Build history of the part. All positions in model axes, mm. A direction names the side the tool comes from. Round coordinates to 2 decimals unless told otherwise and drop trailing zeros. Write each loop counter-clockwise with the first axis right and the second up, starting at its lowest first coordinate (ties: lowest second). Pieces come first, ordered by that corner, then holes.
Item 1: Wall check: probe 1 along X at (y, z) = (0, 5.75); probe 2 along Y at (x, z) = (-60, 25.5); probe 3 along Z at (x, y) = (30, -40.5). Give the ranges that are in metal, low to high.
Item 2: Mould opens along Y. For faces 1 (the flat face through (6.5, -0.2, 10)), 2 (the flat face through (-80, 0, 15)), 3 (the cylindrical face through (73.986, -44.297, 15.21)) say: +Y half, -Y half, draft (parallel to the pull), parting line (faces both ways), or undercut.
Item 3: Band-saw the part on C-C, the plane z = 3. Write the cut outline in (x, y).
Item 4: Band-saw the part on D-D, the plane y = -41.5. Write the cut outline in (x, z).
Item 5: Drop flat-ended pins along their axis: pin 1 Ø6.5 at (x, y) = (39, 2) entering from +Z; pin 2 Ø7.5 at (x, y) = (-60, 0) entering from -Z; pin 3 Ø7.5 at (x, y) = (40, 0) entering from +Z; pin 4 Ø1 at (x, z) = (9.5, 15) entering from +Y. Give the stop position or say it passes through.
Item 6: Band-saw the part on A-A, the plane x = 0. Write the cut outline in (y, z).
Item 7: Band-saw the part on B-B, the plane z = 15.75. Write the cut outline in (x, y), then the cut area to 3 significant figures.
Item 8: 3-axis set-ups, long thin cutter, end or side, ignore diameter. For faces 4 (the flat face through (-60, 6.55, 4)), 5 (the cylindrical face through (-0.8, 21.8, 20.1)), 6 (the cylindrical face through (44.006, 1.262, 20.14)): which of +Z, -Z, +X, -X, +Y, -Y reach the whole face in a straight line?
```python
from build123d import *

# Parameters (mm, degrees)
SKETCH_W        = 160
SKETCH_H        = 100
PAD_DEPTH       = 30
SKETCH001_R     = 6
SKETCH001_R_2   = 4.2
POCKET_DEPTH    = 30
POCKET001_DEPTH = 8
SKETCH003_R     = 15
POCKET002_DEPTH = 10
FILLET_R        = 20
POCKET003_DEPTH = 20
FILLET001_R     = 20
FILLET002_R     = 20
FILLET003_R     = 20
SKETCH006_R     = 4.2
POCKET004_DEPTH = 20


with BuildPart() as part:
    # Sketch → Pad (new body)
    with BuildSketch(Plane.XY):
        Rectangle(SKETCH_W, SKETCH_H)
    extrude(amount=PAD_DEPTH)

    # Sketch001 (on Face6 of Pad) → Pocket (cut)
    with BuildSketch(Plane.XY.offset(30)):
        Circle(SKETCH001_R)
        with Locations((60, 0)):
            Circle(SKETCH001_R_2)
        with Locations((-60, 0)):
            Circle(SKETCH001_R_2)
    extrude(amount=-POCKET_DEPTH, mode=Mode.SUBTRACT)

    # Sketch002 (on Face4 of Pocket) → Pocket001 (cut)
    with BuildSketch(Plane(origin=(0, 0, 0), x_dir=(1, 0, 0), z_dir=(0, 0, -1))):
        Polygon((-52.436711, 0), (-56.218356, 6.55), (-63.781644, 6.55), (-67.563289, 0), (-63.781644, -6.55), (-56.218356, -6.55), align=None)
        Polygon((67.563289, 0), (63.781644, 6.55), (56.218356, 6.55), (52.436711, 0), (56.218356, -6.55), (63.781644, -6.55), align=None)
    extrude(amount=-POCKET001_DEPTH, mode=Mode.SUBTRACT)

    # Sketch003 (on Face4 of Pocket001) → Pocket002 (cut)
    with BuildSketch(Plane(origin=(0, 0, 0), x_dir=(1, 0, 0), z_dir=(0, 0, -1))):
        Circle(SKETCH003_R)
    extrude(amount=-POCKET002_DEPTH, mode=Mode.SUBTRACT)

    # Fillet
    fillet_edges = [part.edges().sort_by_distance(p)[0] for p in [
        (-80, 50, 15),
    ]]
    fillet(fillet_edges, radius=FILLET_R)

    # Sketch004 → Pocket003 (cut)
    with BuildSketch(Plane.XY.offset(30)):
        with BuildLine():
            ThreePointArc((-45, 50), (0, 21.794495), (45, 50))
            Line((-45, 50), (45, 50))
        make_face()
        with BuildLine():
            ThreePointArc((45, -50), (0, -21.794495), (-45, -50))
            Line((-45, -50), (45, -50))
        make_face()
    extrude(amount=-POCKET003_DEPTH, mode=Mode.SUBTRACT)

    # Fillet001
    fillet001_edges = [part.edges().sort_by_distance(p)[0] for p in [
        (80, -50, 15),
    ]]
    fillet(fillet001_edges, radius=FILLET001_R)

    # Fillet002
    fillet002_edges = [part.edges().sort_by_distance(p)[0] for p in [
        (80, 50, 15),
    ]]
    fillet(fillet002_edges, radius=FILLET002_R)

    # Fillet003
    fillet003_edges = [part.edges().sort_by_distance(p)[0] for p in [
        (-80, -50, 15),
    ]]
    fillet(fillet003_edges, radius=FILLET003_R)

    # Sketch006 (on Face23 of Fillet003) → Pocket004 (cut)
    with BuildSketch(Plane.XY.offset(30)):
        with Locations((-40, 0)):
            Circle(SKETCH006_R)
        with Locations((40, 0)):
            Circle(SKETCH006_R)
    extrude(amount=-POCKET004_DEPTH, mode=Mode.SUBTRACT)


solid = part.part
```
Results:
1. probe 1: x = -80 to -67.56, -52.44 to -15, 15 to 52.44, 67.56 to 80
1. probe 2: y = -50 to -4.2, 4.2 to 50
1. probe 3: z = 0 to 10
2. face 1: undercut
2. face 2: draft
2. face 3: -Y half
3. outline: (-80, -30) arc R20 ccw to (-60, -50) - (60, -50) arc R20 ccw to (80, -30) - (80, 30) arc R20 ccw to (60, 50) - (-60, 50) arc R20 ccw to (-80, 30) - close; hole (-67.56, 0) - (-63.78, -6.55) - (-56.22, -6.55) - (-52.44, 0) - (-56.22, 6.55) - (-63.78, 6.55) - close; hole circle Ø30 at (0, 0); hole (52.44, 0) - (56.22, -6.55) - (63.78, -6.55) - (67.56, 0) - (63.78, 6.55) - (56.22, 6.55) - close
4. outline: (-76.36, 0) - (76.36, 0) - (76.36, 30) - (39.78, 30) - (39.78, 10) - (-39.78, 10) - (-39.78, 30) - (-76.36, 30) - close
5. pin 1: stops at z = 30
5. pin 2: passes through
5. pin 3: stops at z = 10
5. pin 4: stops at y = 22.8
6. outline: (-50, 0) - (-15, 0) - (-15, 10) - (-6, 10) - (-6, 30) - (-21.79, 30) - (-21.79, 10) - (-50, 10) - close; (6, 10) - (15, 10) - (15, 0) - (50, 0) - (50, 10) - (21.79, 10) - (21.79, 30) - (6, 30) - close
7. outline: (-80, -30) arc R20 ccw to (-60, -50) - (-45, -50) arc R50 cw to (45, -50) - (60, -50) arc R20 ccw to (80, -30) - (80, 30) arc R20 ccw to (60, 50) - (45, 50) arc R50 cw to (-45, 50) - (-60, 50) arc R20 ccw to (-80, 30) - close; hole circle Ø8.4 at (-60, 0); hole circle Ø8.4 at (-40, 0); hole circle Ø12 at (0, 0); hole circle Ø8.4 at (40, 0); hole circle Ø8.4 at (60, 0)
7. area: 11,700 mm2
8. face 4: -Z
8. face 5: +Z, +Y
8. face 6: +Z
